Verification items for the finished model (mm, model axes). A direction names the side the tool comes from. Give positions to 0.01 mm unless a question says otherwise; leave off trailing zeros. Loops run counter-clockwise (first coordinate to the right, second up) from the corner with the lowest first, then second, coordinate; pieces in that order, holes last. Notation, with made-up numbers: (0.25, 54.25) - (15.25, 54.25) arc R10 ccw to (15.25, 60.25) - close; hole circle Ø10 at (-28.75, -26). An arc over 180 degrees is marked (long way). Put each result on its own line as item: value. Start each with the question number.
```python
from build123d import *

# Parameters (mm, degrees)
SKETCH1_W           = 25.4
SKETCH1_H           = 50.8
BOSS_EXTRUDE1_DEPTH = 6.35
SKETCH2_W           = 44.45
SKETCH2_H           = 7.62
BOSS_EXTRUDE2_DEPTH = 25.4
FILLET1_R           = 12.7
SKETCH3_R           = 3.429
CUT_EXTRUDE1_DEPTH  = 6.35
SKETCH4_R           = 1.8
CUT_EXTRUDE2_DEPTH  = 7.62


with BuildPart() as part:
    # Sketch1 → Boss-Extrude1 (new body)
    with BuildSketch(Plane.XY):
        with Locations((12.7, 25.4)):
            Rectangle(SKETCH1_W, SKETCH1_H)
    extrude(amount=BOSS_EXTRUDE1_DEPTH)

    # Sketch2 → Boss-Extrude2 (add)
    with BuildSketch(Plane(origin=(25.4, 0, 0), x_dir=(0, 0, -1), z_dir=(1, 0, 0))):
        with Locations((-28.575, 3.81)):
            Rectangle(SKETCH2_W, SKETCH2_H)
    extrude(amount=-BOSS_EXTRUDE2_DEPTH)

    # Fillet1
    fillet1_edges = [part.edges().sort_by_distance(p)[0] for p in [
        (12.7, 7.62, 6.35),
    ]]
    fillet(fillet1_edges, radius=FILLET1_R)

    # Sketch3 → Cut-Extrude1 (cut)
    with BuildSketch(Plane.XY.offset(6.35)):
        with Locations((12.7, 44.45)):
            Circle(SKETCH3_R)
        with Locations((12.7, 26.67)):
            Circle(SKETCH3_R)
    extrude(amount=-CUT_EXTRUDE1_DEPTH, mode=Mode.SUBTRACT)

    # Sketch4 → Cut-Extrude2 (cut)
    with BuildSketch(Plane(origin=(0, 7.62, 0), x_dir=(1, 0, 0), z_dir=(0, 1, 0))):
        with Locations(Location((12.7, -25.4, 0), (0, 0, 270))):
            Circle(SKETCH4_R)
        with Locations(Location((22.225, -34.925, 0), (0, 0, 270))):
            Circle(SKETCH4_R)
        with Locations(Location((12.7, -44.45, 0), (0, 0, 270))):
            Circle(SKETCH4_R)
        with Locations(Location((3.175, -34.925, 0), (0, 0, 270))):
            Circle(SKETCH4_R)
    extrude(amount=-CUT_EXTRUDE2_DEPTH, mode=Mode.SUBTRACT)


solid = part.part
```
1) Section check B-B, the plane y = 44.45. Enter the section's corners in (x, z), plus the area to 3 significant figures.
2) Draft check along X on faces 3 (the face through (20.63, 3.86, 35.76)), 4 (the face through (11.605, 3.863, 23.972)), 5 (the face through (0, 9, 12)), 6 (the face through (13, 50.8, 3)). Enter one of: pulls with the +X half, pulls with the -X half, needs draft (parallel to the pull), parting line crosses it, or undercut.
3) Section check D-D, the plane z = 4.5. Enter the section's corners in (x, y).
4) Section check C-C, the plane x = 12.7. Enter the section's corners in (y, z).
5) Section check A-A, the plane z = 25.4. Enter the section's corners in (x, y).
6) Scan lines: line 1 along Y through (x, z) = (12.7, 2.5); line 2 along X through (y, z) = (6.5, 44.5); line 3 along Z through (x, y) = (7.5, 33). Record each from-to range of solid material in increasing order. Write a range as from..to.
7) Depth check by flat-ended pin: P1, Ø7.5, axis at x = 7, z = 36, coming from the +Y side; P2, Ø8, axis at x = 14, y = 37.5, coming from the +Z side; P3, Ø3, axis at x = 3.175, z = 34.925, coming from the -Y side; P4, Ø2, axis at x = 10.5, y = 21, coming from the +Z side. Enter the tip coordinate at first touch or a pass-through.
8) Set-up check for faces 1 (the face through (9.274, 26.821, 3.219)), 2 (the face through (13, 36, 6.35)): record each of +Z, -Z, +X, -X, +Y, -Y from which the full face is reachable in a straight line by a thin tool's end or side.
Results are:
1. outline: (0, 0) - (9.27, 0) - (9.27, 6.35) - (0, 6.35) - close; (16.13, 0) - (25.4, 0) - (25.4, 6.35) - (16.13, 6.35) - close
1. area: 118 mm2
2. face 3: undercut
2. face 4: undercut
2. face 5: pulls with the -X half
2. face 6: needs draft
3. outline: (0, 0) - (25.4, 0) - (25.4, 50.8) - (0, 50.8) - close; hole circle Ø6.86 at (12.7, 26.67); hole circle Ø6.86 at (12.7, 44.45)
4. outline: (0, 0) - (23.24, 0) - (23.24, 6.35) - (20.32, 6.35) arc R12.7 cw to (7.62, 19.05) - (7.62, 23.6) - (0, 23.6) - close; (0, 27.2) - (7.62, 27.2) - (7.62, 42.65) - (0, 42.65) - close; (0, 46.25) - (7.62, 46.25) - (7.62, 50.8) - (0, 50.8) - close; (30.1, 0) - (41.02, 0) - (41.02, 6.35) - (30.1, 6.35) - close; (47.88, 0) - (50.8, 0) - (50.8, 6.35) - (47.88, 6.35) - close
5. outline: (0, 0) - (10.9, 0) - (10.9, 7.62) - (0, 7.62) - close; (14.5, 0) - (25.4, 0) - (25.4, 7.62) - (14.5, 7.62) - close
6. line 1: y = 0..23.24, 30.1..41.02, 47.88..50.8
6. line 2: x = 0..10.9, 14.5..25.4
6. line 3: z = 0..6.35
7. P1: stops at y = 7.62
7. P2: stops at z = 6.35
7. P3: passes through
7. P4: stops at z = 6.35
8. face 1: +Z, -Z
8. face 2: +Z, +X, -X, +Y
